Could you check a few things on this model? Use its own coordinates, in mm. Coordinates: 2 decimals unless noted, no trailing zeros. Order: outer loops, then holes, each group sorted by start corner. A loop starts at its lowest first (then second) coordinate and runs counter-clockwise, first axis right, second up. Notation, with made-up numbers: (73.25, -40) -> (123.25, -40) arc R22 cw to (123.25, -4) -> close; hole circle Ø11 at (-32, 49.5). An arc over 180 degrees is marked (long way). Put each result on its own line as item: value. Start each with the question number.
Q1. If we section it at B-B (y = 0): Please give me the cut outline in (x, z).
Q2. If we section it at A-A (x = 0): Please give me the cut outline in (y, z), and give its area (3 significant figures).
Q3. Please list where these lines run through material, in increasing order: line 1 along Y through (x, z) = (0, 1.2); line 2 along Y through (x, z) = (31, 1.7); line 3 along X through (y, z) = (47.5, 1.3).
Q4. If we section it at D-D (x = 90): Please give me the cut outline in (y, z).
Q5. If we section it at C-C (y = -30): Please give me the cut outline in (x, z), and give its area (3 significant figures).
Q6. Will these pins go through, and if not, where does the flat tip stop? pin 1 (0.6 mm diameter, centred on x = 27, z = 1.5, fed in from +Y); pin 2 (1 mm diameter, centred on x = 6.5, z = 1.5, fed in from +Y); pin 3 (1 mm diameter, centred on x = 11, z = 0.5, fed in from -Y).
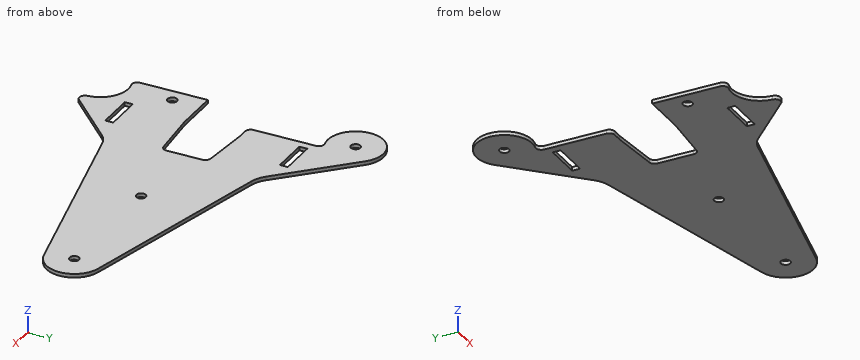
from build123d import *

# Parameters (mm, degrees)
SKETCH1_R           = 2.55
SKETCH1_W           = 20.2
SKETCH1_H           = 4.3
BOSS_EXTRUDE1_DEPTH = 2


with BuildPart() as part:
    # Sketch1 → Boss-Extrude1 (new body)
    with BuildSketch(Plane.XY):
        with BuildLine():
            Line((10.606601718, 79.393398282), (45.794858405, 44.205141595))
            ThreePointArc((45.794858405, 44.205141595), (49.111477563, 41.702351478), (52.987446424, 40.205425828))
            Line((52.987446424, 40.205425828), (162.509181482, 14.606317485))
            ThreePointArc((162.509181482, 14.606317485), (174.095167783, 0), (162.509181482, -14.606317485))
            Line((162.509181482, -14.606317485), (52.987446424, -40.205425828))
            ThreePointArc((52.987446424, -40.205425828), (49.111477563, -41.702351478), (45.794858405, -44.205141595))
            Line((45.794858405, -44.205141595), (45, -45))
            Line((45, -45), (20.188094295, -69.811905705))
            ThreePointArc((20.188094295, -69.811905705), (17.003220161, -70.495733011), (15.072281031, -67.872277826))
            ThreePointArc((15.072281031, -67.872277826), (8.704147834, -56.447922609), (-4.194444444, -54.28105164))
            ThreePointArc((-4.194444444, -54.28105164), (-6.742683116, -53.813165335), (-7.9, -51.495180099))
            Line((-7.9, -51.495180099), (-7.9, -15))
            Line((-7.9, -15), (16.016224064, -15))
            ThreePointArc((16.016224064, -15), (16.147099086, -14.997143929), (16.277724915, -14.988581152))
            Line((16.277724915, -14.988581152), (42.361500851, -12.706250758))
            ThreePointArc((42.361500851, -12.706250758), (44.311843411, -11.744427787), (45.1, -9.717669606))
            Line((45.1, -9.717669606), (45.1, 9.717669606))
            ThreePointArc((45.1, 9.717669606), (44.311843411, 11.744427787), (42.361500851, 12.706250758))
            Line((42.361500851, 12.706250758), (16.277724915, 14.988581152))
            ThreePointArc((16.277724915, 14.988581152), (16.147099086, 14.997143929), (16.016224064, 15))
            Line((16.016224064, 15), (11, 15))
            ThreePointArc((11, 15), (8.878679656, 15.878679656), (8, 18))
            Line((8, 18), (8, 51.495180099))
            ThreePointArc((8, 51.495180099), (6.802775638, 53.89309586), (4.166666667, 54.377116176))
            ThreePointArc((4.166666667, 54.377116176), (-9.013878189, 56.797217756), (-15, 68.786796564))
            ThreePointArc((-15, 68.786796564), (-5.740251485, 82.644989552), (10.606601718, 79.393398282))
        make_face()
        with Locations((159.095167783, 0)):
            Circle(SKETCH1_R, mode=Mode.SUBTRACT)
        with Locations((90, 0)):
            Circle(SKETCH1_R, mode=Mode.SUBTRACT)
        with Locations((0, 68.786796564)):
            Circle(SKETCH1_R, mode=Mode.SUBTRACT)
        with Locations((0, -30)):
            Circle(SKETCH1_R, mode=Mode.SUBTRACT)
        with Locations((22.474619372, 47.05)):
            Rectangle(SKETCH1_W, SKETCH1_H, mode=Mode.SUBTRACT)
        with Locations((22.474619372, -47.05)):
            Rectangle(SKETCH1_W, SKETCH1_H, mode=Mode.SUBTRACT)
    extrude(amount=BOSS_EXTRUDE1_DEPTH)


solid = part.part
The answers:
1. outline: (45.1, 0) -> (87.45, 0) -> (87.45, 2) -> (45.1, 2) -> close; (92.55, 0) -> (156.55, 0) -> (156.55, 2) -> (92.55, 2) -> close; (161.65, 0) -> (174.1, 0) -> (174.1, 2) -> (161.65, 2) -> close
2. outline: (-53.69, 0) -> (-32.55, 0) -> (-32.55, 2) -> (-53.69, 2) -> close; (-27.45, 0) -> (-15, 0) -> (-15, 2) -> (-27.45, 2) -> close; (53.79, 0) -> (66.24, 0) -> (66.24, 2) -> (53.79, 2) -> close; (71.34, 0) -> (83.79, 0) -> (83.79, 2) -> (71.34, 2) -> close
2. area: 117 mm^2
3. line 1: -53.69 to -32.55, -27.45 to -15, 53.79 to 66.24, 71.34 to 83.79
3. line 2: -59 to -49.2, -44.9 to -13.7, 13.7 to 44.9, 49.2 to 59
3. line 3: 8 to 12.37, 32.57 to 42.5
4. outline: (-31.55, 0) -> (-2.55, 0) -> (-2.55, 2) -> (-31.55, 2) -> close; (2.55, 0) -> (31.55, 0) -> (31.55, 2) -> (2.55, 2) -> close
5. outline: (-7.9, 0) -> (-2.55, 0) -> (-2.55, 2) -> (-7.9, 2) -> close; (2.55, 0) -> (96.65, 0) -> (96.65, 2) -> (2.55, 2) -> close
5. area: 199 mm^2
6. pin 1: y = 63.3
6. pin 2: y = 82.53
6. pin 3: y = -59
